Geometry: final body of the model. Coordinates: model frame, mm. A direction names the side the tool comes from. Give positions to 0.01 mm unless a question says otherwise; leave off trailing zeros. Write each loop counter-clockwise with the first axis right and the second up, starting at its lowest first coordinate (ties: lowest second). Pieces come first, ordered by that corner, then holes. Notation, with made-up numbers: (12.25, 65.5) -> (56.25, 65.5) arc R21 cw to (56.25, 69.5) -> close; hole circle Ø7 at (-18, 45.25). An arc over 180 degrees is marked (long way). Answer in a Markdown table with one row per item. Add a question column.
Item 1: Draft query along X for faces 4 (the flat face through (-12.467, 10, -27)), 5 (the flat face through (-20, 14, 5.672)), 6 (the flat face through (-3.577, 14, 7)). Return one class per face: +X half, -X half, draft (parallel to the pull), parting line (faces both ways), or undercut.
Item 2: Material intervals for probe 1 along X at (y, z) = (10, -28.5); probe 2 along Z at (x, y) = (-16.5, 18.5); probe 3 along X at (y, z) = (16.5, -15.5), sorted ascending. Write a range as from..to.
Item 3: First-contact query: P1, Ø1.9, axis at x = -44.5, y = 6.5, coming from the +Z side; P2, Ø5, axis at x = -18.5, y = 14, coming from the -Z side; P3, Ø1.3, axis at y = 15.5, z = -28, coming from the +X side. Flat tips, straight axial feed; report the tip coordinate or a pass-through.
Item 4: Section query C-C on x = -29.5. Output: boundary loops of the cut face in (y, z).
Item 5: Section query A-A on y = 16. Output: boundary loops of the cut face in (x, z), plus the area to 3 significant figures.
Item 6: Access query for faces 1 (the flat face through (-3.577, 14, -27)), 2 (the cylindrical face through (30.49, 1.75, -6.02)), 3 (the flat face through (-43, 7.81, -10)). Directions: +Z, -Z, +X, -X, +Y, -Y. A direction counts if a zero-diameter tool reaches every point of the face in a straight line with its end or side. Return the directions, or none.
Item 7: Section query B-B on z = 2. Output: boundary loops of the cut face in (x, y), plus the area to 3 significant figures.
Item 8: Section query D-D on x = 5.5. Output: boundary loops of the cut face in (y, z).
```python
from build123d import *

# Parameters (mm, degrees)
SKETCH1_W           = 88.138
SKETCH1_H           = 43.688
BOSS_EXTRUDE1_DEPTH = 8.763
CHAMFER1_SIZE       = 2.54
SKETCH2_W           = 2.54
SKETCH2_H           = 12.7
BOSS_EXTRUDE2_DEPTH = 11.43
SKETCH3_W           = 20.32
SKETCH3_H           = 3.81
BOSS_EXTRUDE3_DEPTH = 7.62
CHAMFER2_SIZE       = 2.54
SKETCH4_W           = 12.7
SKETCH4_H           = 2.032
CUT_EXTRUDE1_DEPTH  = 50.8
CUT_EXTRUDE2_DEPTH  = 3.556
CHAMFER3_SIZE       = 6.35


with BuildPart() as part:
    # Sketch1 → Boss-Extrude1 (new body)
    with BuildSketch(Plane(origin=(0, 0, 0), x_dir=(1, 0, 0), z_dir=(0, 1, 0))):
        with Locations((1.121860858, 10.456938882)):
            Rectangle(SKETCH1_W, SKETCH1_H)
    extrude(amount=BOSS_EXTRUDE1_DEPTH)

    # Chamfer1
    chamfer1_edges = [part.edges().sort_by_distance(p)[0] for p in [
        (45.190860858, 8.763, -10.456938882),
        (1.121860858, 8.763, -32.300938882),
        (-42.947139142, 8.763, -10.456938882),
        (1.121860858, 8.763, 11.387061118),
    ]]
    chamfer(chamfer1_edges, length=CHAMFER1_SIZE)

    # Sketch2 → Boss-Extrude2 (add)
    with BuildSketch(Plane(origin=(0, 8.763, 0), x_dir=(1, 0, 0), z_dir=(0, 1, 0))):
        Polygon((-37.867139142, 28.617938882), (-35.327139142, 28.617938882), (-3.577139142, 28.617938882), (-3.577139142, 26.077938882), (-35.327139142, 26.077938882), (-35.327139142, -5.672061118), (-3.577139142, -5.672061118), (-3.577139142, -8.212061118), (-35.327139142, -8.212061118), (-37.867139142, -8.212061118), align=None)
        with Locations((24.362860858, 10.710938882)):
            Rectangle(SKETCH2_W, SKETCH2_H)
    extrude(amount=BOSS_EXTRUDE2_DEPTH)

    # Sketch3 → Boss-Extrude3 (add)
    with BuildSketch(Plane.ZY.offset(37.867139142)):
        with Locations((-9.567938882, 5.9055)):
            Rectangle(SKETCH3_W, SKETCH3_H)
    extrude(amount=BOSS_EXTRUDE3_DEPTH)

    # Chamfer2
    chamfer2_edges = [part.edges().sort_by_distance(p)[0] for p in [
        (-45.487139142, 4.0005, -9.567938882),
    ]]
    chamfer(chamfer2_edges, length=CHAMFER2_SIZE - 0.0001)  # a hair under: the kernel refuses the full size

    # Sketch4 → Cut-Extrude1 (cut)
    with BuildSketch(Plane.XY.offset(8.212061118)):
        with Locations((-18.817139142, 9.779)):
            Rectangle(SKETCH4_W, SKETCH4_H)
    extrude(amount=-CUT_EXTRUDE1_DEPTH, mode=Mode.SUBTRACT)

    # Sketch5 → Cut-Extrude2 (cut)
    with BuildSketch(Plane.XZ):
        with BuildLine():
            Line((35.030860858, -4.106938882), (45.190860858, -4.106938882))
            Line((45.190860858, -4.106938882), (45.190860858, -16.806938882))
            Line((45.190860858, -16.806938882), (45.190860858, -32.300938882))
            add(Edge.make_bspline(
                [(28.680860858, -10.456938882), (28.680860858, -32.300938882), (45.190860858, -32.300938882)],
                knots=[4.71238898, 4.71238898, 4.71238898, 6.283185307, 6.283185307, 6.283185307], degree=2, weights=[1, 0.707106781, 1]))
            ThreePointArc((28.680860858, -10.456938882), (30.540732798, -5.966810821), (35.030860858, -4.106938882))
        make_face()
    extrude(amount=-CUT_EXTRUDE2_DEPTH, mode=Mode.SUBTRACT)

    # Chamfer3
    chamfer3_edges = [part.edges().sort_by_distance(p)[0] for p in [
        (25.632860858, 8.763, -10.710938882),
    ]]
    chamfer(chamfer3_edges, length=CHAMFER3_SIZE)


solid = part.part
```
Findings below:
| question | item | result |
|---|---|---|
| 1 | face 4 | undercut |
| 1 | face 5 | draft |
| 1 | face 6 | +X half |
| 2 | probe 1 | x = -37.87..-25.17, -12.47..-3.58 |
| 2 | probe 2 | z = -28.62..-26.08, 5.67..8.21 |
| 2 | probe 3 | x = -37.87..-35.33, 23.09..25.63 |
| 3 | P1 | stops at z = 0.59 |
| 3 | P2 | stops at z = -28.62 |
| 3 | P3 | stops at x = -3.58 |
| 4 | outline | (0, -32.3) -> (6.22, -32.3) -> (8.76, -29.76) -> (8.76, -28.62) -> (20.19, -28.62) -> (20.19, -26.08) -> (8.76, -26.08) -> (8.76, 5.67) -> (20.19, 5.67) -> (20.19, 8.21) -> (8.76, 8.21) -> (8.76, 8.85) -> (6.22, 11.39) -> (0, 11.39) -> close |
| 5 | outline | (-37.87, -28.62) -> (-3.58, -28.62) -> (-3.58, -26.08) -> (-35.33, -26.08) -> (-35.33, 5.67) -> (-3.58, 5.67) -> (-3.58, 8.21) -> (-37.87, 8.21) -> close; (23.09, -17.06) -> (25.63, -17.06) -> (25.63, -4.36) -> (23.09, -4.36) -> close |
| 5 | area | 287 mm^2 |
| 6 | face 1 | +Z, -Z, +X, +Y |
| 6 | face 2 | +X, -Y |
| 6 | face 3 | +Z, -Z, -X, +Y |
| 7 | outline | (-42.95, 0) -> (45.19, 0) -> (45.19, 6.22) -> (42.65, 8.76) -> (-35.33, 8.76) -> (-35.33, 20.19) -> (-37.87, 20.19) -> (-37.87, 8.76) -> (-40.41, 8.76) -> (-42.95, 6.22) -> close |
| 7 | area | 795 mm^2 |
| 8 | outline | (0, -32.3) -> (6.22, -32.3) -> (8.76, -29.76) -> (8.76, 8.85) -> (6.22, 11.39) -> (0, 11.39) -> close |
